Part print with two shaded views. Sizes in mm from the minimum x, y, z corner. A direction names the side the tool comes from. Coordinates: 2 decimals unless noted, no trailing zeros. Loops run counter-clockwise (first coordinate to the right, second up) from the corner with the lowest first, then second, coordinate; pieces in that order, holes last. Notation, with made-up numbers: (-18, -24) - (16, -24) arc R16 ccw to (16, 6) - close; hole circle Ø4 at (30, -26.75). An arc over 180 degrees is marked (long way). Write each question's results on one line, items separated by ' | '. Start each with the question number.
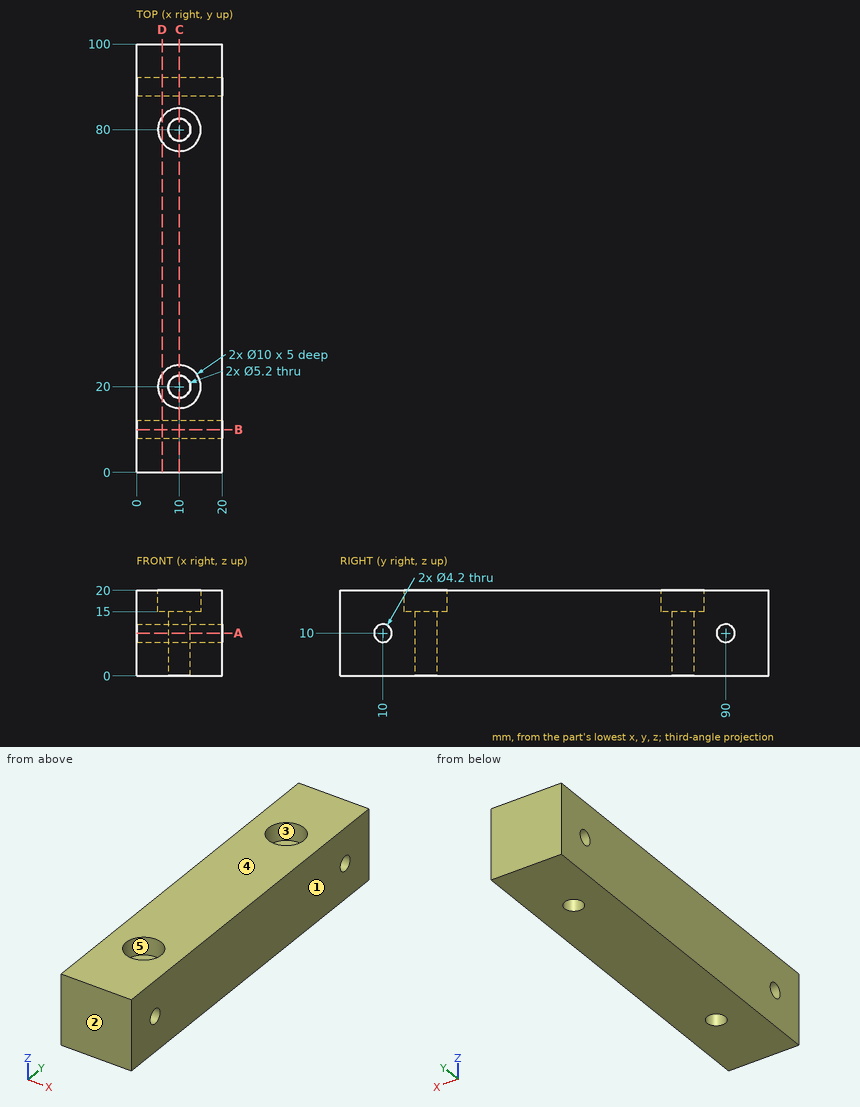
Q1. Pin check, flat tips, straight feed: pin 1 (4 mm diameter, centred on y = 90, z = 10, fed in from -X); pin 2 (8 mm diameter, centred on x = 10, y = 80, fed in from +Z). Stop position of each tip, or through.
Q2. Mould opens along Y. For the marked faces 1, 2 and 3 say: +Y half, -Y half, draft (parallel to the pull), parting line (faces both ways), or undercut.
Q3. Cut at A-A (z = 10). List the corners of the cut face in (x, y).
Q4. Cut at C-C (x = 10). List the corners of the cut face in (y, z).
Q5. Cut at D-D (x = 6). List the corners of the cut face in (y, z), and give its area (3 significant figures).
Q6. Drill centre lines: L1, parallel to Y at x = 10, z = 16.95; L2, parallel to Y at x = 10, z = 3.5; L3, parallel to Z at x = 12, y = 82. Where is each one in solid material? Low to high. Write a range as from..to.
Q7. Which spindle directions (+Z, -Z, +X, -X, +Y, -Y) get a long thin tool onto all of the face, cutting with end or side? Do the marked faces 4 and 5. Say none if no direction does.
Q8. Cut at B-B (y = 10). List the corners of the cut face in (x, z).
Check result:
1) pin 1: through | pin 2: z = 15
2) face 1: draft | face 2: -Y half | face 3: undercut
3) outline: (0, 0) - (20, 0) - (20, 7.9) - (0, 7.9) - close; (0, 12.1) - (20, 12.1) - (20, 87.9) - (0, 87.9) - close; (0, 92.1) - (20, 92.1) - (20, 100) - (0, 100) - close; hole circle Ø5.2 at (10, 20); hole circle Ø5.2 at (10, 80)
4) outline: (0, 0) - (17.4, 0) - (17.4, 15) - (15, 15) - (15, 20) - (0, 20) - close; (22.6, 0) - (77.4, 0) - (77.4, 15) - (75, 15) - (75, 20) - (25, 20) - (25, 15) - (22.6, 15) - close; (82.6, 0) - (100, 0) - (100, 20) - (85, 20) - (85, 15) - (82.6, 15) - close; hole circle Ø4.2 at (10, 10); hole circle Ø4.2 at (90, 10)
5) outline: (0, 0) - (100, 0) - (100, 20) - (83, 20) - (83, 15) - (77, 15) - (77, 20) - (23, 20) - (23, 15) - (17, 15) - (17, 20) - (0, 20) - close; hole circle Ø4.2 at (10, 10); hole circle Ø4.2 at (90, 10) | area: 1,910 mm²
6) L1: 0..15, 25..75, 85..100 | L2: 0..17.4, 22.6..77.4, 82.6..100 | L3: 0..15
7) face 4: +Z, +X, -X, +Y, -Y | face 5: +Z
8) outline: (0, 0) - (20, 0) - (20, 7.9) - (0, 7.9) - close; (0, 12.1) - (20, 12.1) - (20, 20) - (0, 20) - close
